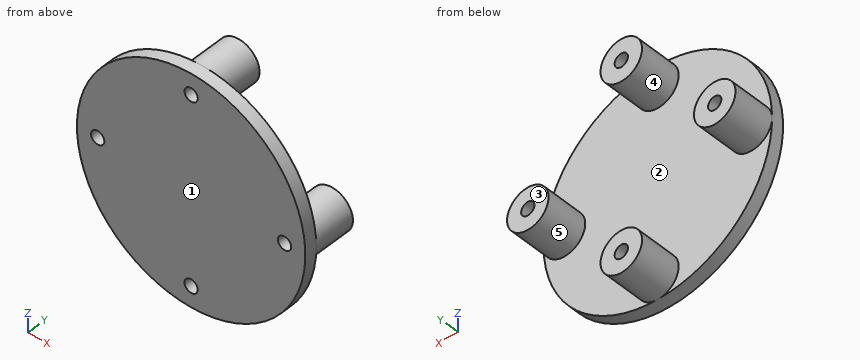
```python
from build123d import *

# Parameters (mm, degrees)
SKETCH1_R           = 27.5
BOSS_EXTRUDE1_DEPTH = 3
SKETCH3_R           = 5
BOSS_EXTRUDE2_DEPTH = 10
SKETCH4_R           = 1.6
CUT_EXTRUDE1_DEPTH  = 42.006097108


with BuildPart() as part:
    # Sketch1 → Boss-Extrude1 (new body)
    with BuildSketch(Plane(origin=(0, 0, 0), x_dir=(1, 0, 0), z_dir=(0, 1, 0))):
        with Locations(Location((0, 0, 0), (0, 0, 270))):
            Circle(SKETCH1_R)
    extrude(amount=BOSS_EXTRUDE1_DEPTH)

    # Sketch3 → Boss-Extrude2 (add)
    with BuildSketch(Plane(origin=(0, 3, 0), x_dir=(1, 0, 0), z_dir=(0, 1, 0))):
        with Locations(Location((0, 22.5, 0), (0, 0, 89.999599385))):
            Circle(SKETCH3_R)
        with Locations(Location((22.5, 0, 0), (0, 0, 359.999599385))):
            Circle(SKETCH3_R)
        with Locations(Location((0, -22.5, 0), (0, 0, 269.999599385))):
            Circle(SKETCH3_R)
        with Locations(Location((-22.5, 0, 0), (0, 0, 179.999599385))):
            Circle(SKETCH3_R)
    extrude(amount=BOSS_EXTRUDE2_DEPTH)

    # Sketch4 → Cut-Extrude1 (cut, through all)
    with BuildSketch(Plane(origin=(0, 13, 0), x_dir=(1, 0, 0), z_dir=(0, 1, 0))):
        with Locations(Location((0, 22.5, 0), (0, 0, 270))):
            Circle(SKETCH4_R)
        with Locations(Location((22.5, 0, 0), (0, 0, 270))):
            Circle(SKETCH4_R)
        with Locations(Location((0, -22.5, 0), (0, 0, 270))):
            Circle(SKETCH4_R)
        with Locations(Location((-22.5, 0, 0), (0, 0, 270))):
            Circle(SKETCH4_R)
    extrude(amount=-CUT_EXTRUDE1_DEPTH, mode=Mode.SUBTRACT)


solid = part.part
```
Part model, mm, in its own coordinate system. Face numbers are marked on the shaded views. A direction names the side the tool comes from. Coordinates: 2 decimals unless noted, no trailing zeros. Write each loop counter-clockwise with the first axis right and the second up, starting at its lowest first coordinate (ties: lowest second). Pieces come first, ordered by that corner, then holes.
Item 1: Pin check, flat tips, straight feed: pin 1 (6 mm diameter, centred on y = 3.5, z = -11.5, fed in from -X); pin 2 (2.5 mm diameter, centred on x = -22.5, z = 0, fed in from -Y); pin 3 (2 mm diameter, centred on x = 0, z = -6, fed in from +Y); pin 4 (5 mm diameter, centred on y = 3, z = -11, fed in from +X). Stop position of each tip, or through.
Item 2: Slice it at B-B (x = -22.5). Write the cut outline in (y, z).
Item 3: Mould opens along Z. For the marked faces 3, 4 and 5 say: released by +Z, released by -Z, zero draft, split by the parting line, or undercut.
Item 4: Slice it at D-D (x = -2.5). Write the cut outline in (y, z).
Item 5: Which spindle directions (+Z, -Z, +X, -X, +Y, -Y) get a long thin tool onto all of the face, cutting with end or side? Do the marked faces 1 and 2. Say none if no direction does.
Item 6: Probe line 1 (X direction, y = 7.5, z = 0); line 2 (X direction, y = 9.5, z = 22.5); line 3 (X direction, y = 0.5, z = 1). List the from-to ranges inside material, lowest first.
Item 7: Slice it at A-A (y = 10). Write the cut outline in (x, z), and give its area (3 significant figures).
Item 8: Slice it at C-C (z = 22.5). Write the cut outline in (x, y), and give its area (3 significant figures).
Results found:
1. pin 1: stops at x = -26.14
1. pin 2: passes through
1. pin 3: stops at y = 3
1. pin 4: stops at x = 26.15
2. outline: (0, -15.81) - (3, -15.81) - (3, -5) - (13, -5) - (13, -1.6) - (0, -1.6) - close; (0, 1.6) - (13, 1.6) - (13, 5) - (3, 5) - (3, 15.81) - (0, 15.81) - close
3. face 3: zero draft
3. face 4: undercut
3. face 5: split by the parting line
4. outline: (0, -27.39) - (3, -27.39) - (3, -26.83) - (13, -26.83) - (13, -18.17) - (3, -18.17) - (3, 18.17) - (13, 18.17) - (13, 26.83) - (3, 26.83) - (3, 27.39) - (0, 27.39) - close
5. face 1: +Z, -Z, +X, -X, -Y
5. face 2: +Y
6. line 1: x = -27.5 to -24.1, -20.9 to -17.5, 17.5 to 20.9, 24.1 to 27.5
6. line 2: x = -5 to -1.6, 1.6 to 5
6. line 3: x = -27.48 to -23.75, -21.25 to 21.25, 23.75 to 27.48
7. outline: circle Ø10 at (-22.5, 0); circle Ø10 at (0, -22.5); circle Ø10 at (0, 22.5); circle Ø10 at (22.5, 0); hole circle Ø3.2 at (-22.5, 0); hole circle Ø3.2 at (0, -22.5); hole circle Ø3.2 at (0, 22.5); hole circle Ø3.2 at (22.5, 0)
7. area: 282 mm2
8. outline: (-15.81, 0) - (-1.6, 0) - (-1.6, 13) - (-5, 13) - (-5, 3) - (-15.81, 3) - close; (1.6, 0) - (15.81, 0) - (15.81, 3) - (5, 3) - (5, 13) - (1.6, 13) - close
8. area: 153 mm2
